from build123d import *

# Parameters (mm, degrees)
SKETCH_10_R         = 1.7
EXTRUDE_5_DEPTH     = 6
EXTRUDE_6_DEPTH     = 1.2
EXTRUDE_START       = -7.1
EXTRUDE_7_DEPTH     = 7.1
CUT_EXTRUDE_3_REACH = 209.716
CUT_EXTRUDE_4_DEPTH = 0.4
EXTRUDE_START_2     = 6
EXTRUDE_8_DEPTH     = 6
SKETCH_15_R         = 2
SKETCH_15_R_2       = 1
CUT_EXTRUDE_5_DEPTH = 1.2


with BuildPart() as part:
    # 草图10 → 凸台-拉伸5 (new body)
    with BuildSketch(Plane(origin=(0, 0, 53.48299881), x_dir=(-1, 0, 0), z_dir=(0, 0, -1))):
        with BuildLine():
            ThreePointArc((9.233430205, 182.453191023), (7.421209024, 186.828279976), (3.04612007, 188.640501158))
            Line((3.04612007, 188.640501158), (-46.95397899, 188.640501158))
            ThreePointArc((-46.95397899, 188.640501158), (-51.329067943, 186.828279976), (-53.141289124, 182.453191023))
            Line((-53.141289124, 182.453191023), (-53.141289124, 152.453132603))
            ThreePointArc((-53.141289124, 152.453132603), (-51.329067943, 148.078043649), (-46.95397899, 146.265822468))
            Line((-46.95397899, 146.265822468), (3.04612007, 146.265822468))
            ThreePointArc((3.04612007, 146.265822468), (7.421209024, 148.078043649), (9.233430205, 152.453132603))
            Line((9.233430205, 152.453132603), (9.233430205, 182.453191023))
        make_face()
        with BuildLine():
            ThreePointArc((0.54612261, 185.453196103), (1.717695486, 182.624768978), (4.54612261, 181.453196103))
            Line((4.54612261, 181.453196103), (8.233430205, 181.453196103))
            Line((8.233430205, 181.453196103), (8.233430205, 153.453127523))
            Line((8.233430205, 153.453127523), (4.54612261, 153.453127523))
            ThreePointArc((4.54612261, 153.453127523), (1.717695486, 152.281554648), (0.54612261, 149.453127523))
            Line((0.54612261, 149.453127523), (0.54612261, 147.265822468))
            Line((0.54612261, 147.265822468), (-45.95398153, 147.265822468))
            Line((-45.95398153, 147.265822468), (-45.95398153, 150.953127523))
            ThreePointArc((-45.95398153, 150.953127523), (-46.686214577, 152.720894476), (-48.45398153, 153.453127523))
            Line((-48.45398153, 153.453127523), (-52.141289124, 153.453127523))
            Line((-52.141289124, 153.453127523), (-52.141289124, 180.953183403))
            Line((-52.141289124, 180.953183403), (-48.45399423, 180.953183403))
            ThreePointArc((-48.45399423, 180.953183403), (-46.332673886, 181.831863059), (-45.45399423, 183.953183403))
            Line((-45.45399423, 183.953183403), (-45.45399423, 187.640501158))
            Line((-45.45399423, 187.640501158), (0.54612261, 187.640501158))
            Line((0.54612261, 187.640501158), (0.54612261, 185.453196103))
        make_face(mode=Mode.SUBTRACT)
        with Locations((4.54610737, 183.953163083)):
            Circle(SKETCH_10_R, mode=Mode.SUBTRACT)
        with Locations((-48.45399423, 183.953183403)):
            Circle(SKETCH_10_R, mode=Mode.SUBTRACT)
        with Locations((-48.45399423, 150.953140223)):
            Circle(SKETCH_10_R, mode=Mode.SUBTRACT)
        with Locations((4.54610737, 150.953160543)):
            Circle(SKETCH_10_R, mode=Mode.SUBTRACT)
    extrude(amount=EXTRUDE_5_DEPTH)

    # 草图11 → 凸台-拉伸6 (add)
    with BuildSketch(Plane(origin=(0, 0, 47.48299881), x_dir=(-1, 0, 0), z_dir=(0, 0, -1))):
        with BuildLine():
            Line((9.233430205, 152.453132603), (9.233430205, 182.453191023))
            ThreePointArc((9.233430205, 182.453191023), (7.421209024, 186.828279976), (3.04612007, 188.640501158))
            Line((3.04612007, 188.640501158), (-46.95397899, 188.640501158))
            ThreePointArc((-46.95397899, 188.640501158), (-51.329067943, 186.828279976), (-53.141289124, 182.453191023))
            Line((-53.141289124, 182.453191023), (-53.141289124, 152.453132603))
            ThreePointArc((-53.141289124, 152.453132603), (-51.329067943, 148.078043649), (-46.95397899, 146.265822468))
            Line((-46.95397899, 146.265822468), (3.04612007, 146.265822468))
            ThreePointArc((3.04612007, 146.265822468), (7.421209024, 148.078043649), (9.233430205, 152.453132603))
        make_face()
    extrude(amount=EXTRUDE_6_DEPTH)

    # 草图10<4> → 凸台-拉伸7 (add)
    with BuildSketch(Plane(origin=(0, 0, 53.48299881), x_dir=(-1, 0, 0), z_dir=(0, 0, -1)).offset(EXTRUDE_START)):
        with BuildLine():
            Line((9.233430205, 152.453132603), (9.233430205, 182.453191023))
            ThreePointArc((9.233430205, 182.453191023), (7.421209024, 186.828279976), (3.04612007, 188.640501158))
            Line((3.04612007, 188.640501158), (-46.95397899, 188.640501158))
            ThreePointArc((-46.95397899, 188.640501158), (-51.329067943, 186.828279976), (-53.141289124, 182.453191023))
            Line((-53.141289124, 182.453191023), (-53.141289124, 152.453132603))
            ThreePointArc((-53.141289124, 152.453132603), (-51.329067943, 148.078043649), (-46.95397899, 146.265822468))
            Line((-46.95397899, 146.265822468), (3.04612007, 146.265822468))
            ThreePointArc((3.04612007, 146.265822468), (7.421209024, 148.078043649), (9.233430205, 152.453132603))
        make_face()
        with BuildLine():
            ThreePointArc((8.233430205, 182.453191023), (6.714102243, 186.121173195), (3.04612007, 187.640501158))
            Line((3.04612007, 187.640501158), (-46.95397899, 187.640501158))
            ThreePointArc((-46.95397899, 187.640501158), (-50.621961162, 186.121173195), (-52.141289124, 182.453191023))
            Line((-52.141289124, 182.453191023), (-52.141289124, 152.453132603))
            ThreePointArc((-52.141289124, 152.453132603), (-50.621961162, 148.78515043), (-46.95397899, 147.265822468))
            Line((-46.95397899, 147.265822468), (3.04612007, 147.265822468))
            ThreePointArc((3.04612007, 147.265822468), (6.714102243, 148.78515043), (8.233430205, 152.453132603))
            Line((8.233430205, 152.453132603), (8.233430205, 182.453191023))
        make_face(mode=Mode.SUBTRACT)
    extrude(amount=EXTRUDE_7_DEPTH)

    # 草图12 → 切除-拉伸3 (cut, up to next)
    with BuildSketch(Plane(origin=(53.141289124, 0, 0), x_dir=(0, 0, -1), z_dir=(1, 0, 0)), mode=Mode.PRIVATE) as cut_extrude_3_sk1:
        with BuildLine():
            Line((-57.343049783, 179.450176225), (-55.943049648, 179.450176225))
            ThreePointArc((-55.943049648, 179.450176225), (-55.235942867, 179.157283006), (-54.943049648, 178.450176225))
            Line((-54.943049648, 178.450176225), (-54.943049648, 171.310175849))
            ThreePointArc((-54.943049648, 171.310175849), (-55.235942867, 170.603069068), (-55.943049648, 170.310175849))
            Line((-55.943049648, 170.310175849), (-57.343049783, 170.310175849))
            ThreePointArc((-57.343049783, 170.310175849), (-58.050156564, 170.603069068), (-58.343049783, 171.310175849))
            Line((-58.343049783, 171.310175849), (-58.343049783, 178.450176225))
            ThreePointArc((-58.343049783, 178.450176225), (-58.050156564, 179.157283006), (-57.343049783, 179.450176225))
        make_face()
    cut_extrude_3_tool1 = extrude(cut_extrude_3_sk1.sketch, amount=-CUT_EXTRUDE_3_REACH, mode=Mode.PRIVATE) & part.part
    add(cut_extrude_3_tool1.solids().sort_by_distance((53.141289, 174.880176, 56.64305))[0], mode=Mode.SUBTRACT)

    # 草图13 → 切除-拉伸4 (cut)
    with BuildSketch(Plane(origin=(53.141289124, 0, 0), x_dir=(0, 0, -1), z_dir=(1, 0, 0))):
        with BuildLine():
            Line((-57.143049715, 180.880176037), (-56.143049715, 180.880176037))
            ThreePointArc((-56.143049715, 180.880176037), (-54.375282762, 180.14794299), (-53.643049715, 178.380176037))
            Line((-53.643049715, 178.380176037), (-53.643049715, 171.380176037))
            ThreePointArc((-53.643049715, 171.380176037), (-54.375282762, 169.612409084), (-56.143049715, 168.880176037))
            Line((-56.143049715, 168.880176037), (-57.143049715, 168.880176037))
            ThreePointArc((-57.143049715, 168.880176037), (-58.910816668, 169.612409084), (-59.643049715, 171.380176037))
            Line((-59.643049715, 171.380176037), (-59.643049715, 178.380176037))
            ThreePointArc((-59.643049715, 178.380176037), (-58.910816668, 180.14794299), (-57.143049715, 180.880176037))
        make_face()
    extrude(amount=-CUT_EXTRUDE_4_DEPTH, mode=Mode.SUBTRACT)

    # 草图14 → 凸台-拉伸8 (add)
    with BuildSketch(Plane.XY.offset(47.48299881).offset(EXTRUDE_START_2)):
        with BuildLine():
            ThreePointArc((46.196138585, 152.026507807), (37.131275676, 156.428908647), (46.516064334, 160.100231917))
            ThreePointArc((46.516064334, 160.100231917), (47.708316282, 158.315900782), (48.12697949, 156.211138699))
            ThreePointArc((48.12697949, 156.211138699), (47.878381245, 154.576273637), (47.155059599, 153.089199108))
            ThreePointArc((47.155059599, 153.089199108), (47.779510983, 153.360426732), (48.45398153, 153.453127523))
            Line((48.45398153, 153.453127523), (48.512842608, 153.453127523))
            ThreePointArc((48.512842608, 153.453127523), (48.971587844, 154.79835866), (49.12697949, 156.211138699))
            ThreePointArc((49.12697949, 156.211138699), (36.975612676, 159.422408955), (45.95398153, 150.627133812))
            Line((45.95398153, 150.627133812), (45.95398153, 150.953127523))
            ThreePointArc((45.95398153, 150.953127523), (46.0152721, 151.503305965), (46.196138585, 152.026507807))
        make_face()
    extrude(amount=-EXTRUDE_8_DEPTH)

    # 草图15 → 切除-拉伸5 (cut)
    with BuildSketch(Plane(origin=(0, 0, 46.28299881), x_dir=(-1, 0, 0), z_dir=(0, 0, -1))):
        with Locations((-42.647049867, 156.215638701)):
            Circle(SKETCH_15_R)
        with Locations((-46.426971116, 156.211138699)):
            Circle(SKETCH_15_R_2)
        with Locations((-42.651549869, 159.995559949)):
            Circle(SKETCH_15_R_2)
        with Locations((-38.867128618, 156.220138702)):
            Circle(SKETCH_15_R_2)
        with Locations((-42.642549865, 152.435717452)):
            Circle(SKETCH_15_R_2)
    extrude(amount=-CUT_EXTRUDE_5_DEPTH, mode=Mode.SUBTRACT)


solid = part.part
Geometry: final body of the model. Coordinates: model frame, mm. A direction names the side the tool comes from. Give positions to 0.01 mm unless a question says otherwise; leave off trailing zeros. Order: outer loops, then holes, each group sorted by start corner. A loop starts at its lowest first (then second) coordinate and runs counter-clockwise, first axis right, second up. Notation, with made-up numbers: (1.25, 28) -> (34.25, 28) arc R16 cw to (34.25, 58) -> close; hole circle Ø5 at (-16.75, 42). An arc over 180 degrees is marked (long way). Put each result on its own line as item: value.
Q1. Section C-C, the plane z = 52. Count the separate pieces of the cut face and the enclosed holes in it, then the cut area to 3 significant figures.
Here are the results:
separate pieces: 1
enclosed holes: 6
area: 339 mm^2
Q2. Section B-B, the plane x = 20. Return loops of the section in (y, z).
Here are the results:
outline: (146.27, 46.28) -> (188.64, 46.28) -> (188.64, 60.58) -> (187.64, 60.58) -> (187.64, 47.48) -> (147.27, 47.48) -> (147.27, 60.58) -> (146.27, 60.58) -> close
Q3. Material intervals for L1, parallel to X at y = 163.5, z = 54.5; L2, parallel to Y at x = 18, z = 59.5; L3, parallel to Y at x = 38.5, z = 48, sorted ascending.
Here are the results:
L1: x = -9.23 to -8.23, 52.14 to 53.14
L2: y = 146.27 to 147.27, 187.64 to 188.64
L3: y = 146.27 to 147.27, 151.19 to 152.58, 159.85 to 161.23, 187.64 to 188.64
Q4. Section D-D, the plane y = 167.5. Return loops of the section in (x, z).
Here are the results:
outline: (-9.23, 46.28) -> (53.14, 46.28) -> (53.14, 60.58) -> (52.14, 60.58) -> (52.14, 47.48) -> (-8.23, 47.48) -> (-8.23, 60.58) -> (-9.23, 60.58) -> close
Q5. Draft query along Z for faces 1 (the face through (52.741, 175, 54.6)), 2 (the face through (22, 168, 46.283)), 3 (the face through (47.67, 182.445, 50.525)). Return one class per face: released by +Z, released by -Z, zero draft, split by the parting line, or undercut.
Here are the results:
face 1: undercut
face 2: released by -Z
face 3: zero draft
Q6. Reachability of faces 4 (the face through (48, 151, 47.483)), 5 (the face through (53.141, 168, 54)) from +Z, -Z, +X, -X, +Y, -Y: full face, straight path, thin tool, end or side. Return the list, or none.
Here are the results:
face 4: +Z
face 5: +Z, -Z, +X, +Y, -Y
Q7. Pin query (flat end, axial travel): pin 1 (3 mm diameter, centred on y = 185.5, z = 52, fed in from -X); pin 2 (4 mm diameter, centred on x = -7, z = 49, fed in from -Y); pin 3 (2.5 mm diameter, centred on x = 48, y = 184.5, fed in from +Z); pin 4 (1.2 mm diameter, centred on x = 42.64, y = 152.44, fed in from +Z). Return the tip coordinate at first contact, or that it passes through.
Here are the results:
pin 1: stops at x = -9.04
pin 2: stops at y = 146.58
pin 3: stops at z = 53.48
pin 4: passes through
Q8. Section A-A, the plane y = 176. Return loops of the section in (x, z).
Here are the results:
outline: (-9.23, 46.28) -> (53.14, 46.28) -> (53.14, 53.64) -> (52.74, 53.64) -> (52.74, 54.94) -> (52.14, 54.94) -> (52.14, 47.48) -> (-8.23, 47.48) -> (-8.23, 60.58) -> (-9.23, 60.58) -> close; (52.14, 58.34) -> (52.74, 58.34) -> (52.74, 59.64) -> (53.14, 59.64) -> (53.14, 60.58) -> (52.14, 60.58) -> close
